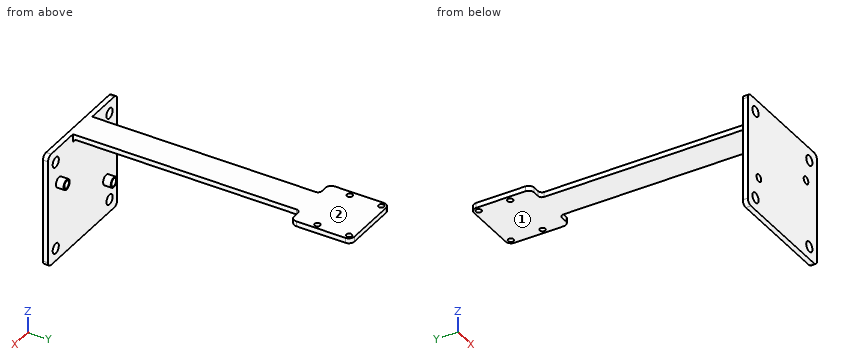
from build123d import *

# Parameters (mm, degrees)
SKETCH1_R           = 1.1
BOSS_EXTRUDE1_DEPTH = 2
FILLET1_R           = 2.2
FILLET2_R           = 2.2
FILLET3_R           = 2.2
FILLET5_R           = 2.2
FILLET6_R           = 1.5
FILLET7_R           = 1.5
SKETCH5_W           = 45
SKETCH5_H           = 45
SKETCH5_R           = 2
BOSS_EXTRUDE4_DEPTH = 2
FILLET17_R          = 2
FILLET18_R          = 2
FILLET19_R          = 2
FILLET20_R          = 2
FILLET21_R          = 1.5
SKETCH7_R           = 2
BOSS_EXTRUDE8_DEPTH = 5
SKETCH10_R          = 1.5
CUT_EXTRUDE4_DEPTH  = 6


with BuildPart() as part:
    # Sketch1 → Boss-Extrude1 (new body)
    with BuildSketch(Plane.XY):
        Polygon((6.25, 0), (6.25, -90), (18.75, -90), (18.75, 0), (25, 0), (25, 23.862), (0, 23.862), (0, 0), align=None)
        with Locations((2, 21.862)):
            Circle(SKETCH1_R, mode=Mode.SUBTRACT)
        with Locations((23, 21.862)):
            Circle(SKETCH1_R, mode=Mode.SUBTRACT)
        with Locations((2, 9.362)):
            Circle(SKETCH1_R, mode=Mode.SUBTRACT)
        with Locations((23, 9.362)):
            Circle(SKETCH1_R, mode=Mode.SUBTRACT)
    extrude(amount=BOSS_EXTRUDE1_DEPTH)

    # Fillet1
    fillet1_edges = [part.edges().sort_by_distance(p)[0] for p in [
        (0, 0, 1),
    ]]
    fillet(fillet1_edges, radius=FILLET1_R)

    # Fillet2
    fillet2_edges = [part.edges().sort_by_distance(p)[0] for p in [
        (0, 23.862, 1),
    ]]
    fillet(fillet2_edges, radius=FILLET2_R)

    # Fillet3
    fillet3_edges = [part.edges().sort_by_distance(p)[0] for p in [
        (25, 23.862, 1),
    ]]
    fillet(fillet3_edges, radius=FILLET3_R)

    # Fillet5
    fillet5_edges = [part.edges().sort_by_distance(p)[0] for p in [
        (25, 0, 1),
    ]]
    fillet(fillet5_edges, radius=FILLET5_R)

    # Fillet6
    fillet6_edges = [part.edges().sort_by_distance(p)[0] for p in [
        (18.75, 0, 1),
    ]]
    fillet(fillet6_edges, radius=FILLET6_R)

    # Fillet7
    fillet7_edges = [part.edges().sort_by_distance(p)[0] for p in [
        (6.25, 0, 1),
    ]]
    fillet(fillet7_edges, radius=FILLET7_R)

    # Sketch5 → Boss-Extrude4 (add)
    with BuildSketch(Plane.XZ.offset(90)):
        with Locations((12.5, -20.5)):
            Rectangle(SKETCH5_W, SKETCH5_H)
        with Locations((-5, -3)):
            Circle(SKETCH5_R, mode=Mode.SUBTRACT)
        with Locations((-5, -38)):
            Circle(SKETCH5_R, mode=Mode.SUBTRACT)
        with Locations((30, -3)):
            Circle(SKETCH5_R, mode=Mode.SUBTRACT)
        with Locations((30, -38)):
            Circle(SKETCH5_R, mode=Mode.SUBTRACT)
    extrude(amount=BOSS_EXTRUDE4_DEPTH)

    # Fillet17
    fillet17_edges = [part.edges().sort_by_distance(p)[0] for p in [
        (35, -91, 2),
    ]]
    fillet(fillet17_edges, radius=FILLET17_R)

    # Fillet18
    fillet18_edges = [part.edges().sort_by_distance(p)[0] for p in [
        (-10, -91, 2),
    ]]
    fillet(fillet18_edges, radius=FILLET18_R)

    # Fillet19
    fillet19_edges = [part.edges().sort_by_distance(p)[0] for p in [
        (-10, -91, -43),
    ]]
    fillet(fillet19_edges, radius=FILLET19_R)

    # Fillet20
    fillet20_edges = [part.edges().sort_by_distance(p)[0] for p in [
        (35, -91, -43),
    ]]
    fillet(fillet20_edges, radius=FILLET20_R)

    # Fillet21
    fillet21_edges = [part.edges().sort_by_distance(p)[0] for p in [
        (12.5, -90, 0),
    ]]
    fillet(fillet21_edges, radius=FILLET21_R)

    # Sketch7 → Boss-Extrude8 (add)
    with BuildSketch(Plane.XZ.offset(92)):
        with Locations((27.85, -12.25)):
            Circle(SKETCH7_R)
        with Locations((-2.85, -28.75)):
            Circle(SKETCH7_R)
    extrude(amount=-BOSS_EXTRUDE8_DEPTH)

    # Sketch10 → Cut-Extrude4 (cut, through all)
    with BuildSketch(Plane(origin=(0, -87, 0), x_dir=(1, 0, 0), z_dir=(0, 1, 0))):
        with Locations((27.85, 12.25)):
            Circle(SKETCH10_R)
        with Locations((-2.85, 28.75)):
            Circle(SKETCH10_R)
    extrude(amount=-CUT_EXTRUDE4_DEPTH, mode=Mode.SUBTRACT)


solid = part.part
Input: part model. Units: mm. Frame: model coordinates. Face numbers are marked on the shaded views. A direction names the side the tool comes from. Give positions to 0.01 mm unless a question says otherwise; leave off trailing zeros. Order: outer loops, then holes, each group sorted by start corner. A loop starts at its lowest first (then second) coordinate and runs counter-clockwise, first axis right, second up.
Q1. Contact query for flat-ended pins moving along their axis: pin 1 Ø1 at (y, z) = (11.5, 1) entering from +X; pin 2 Ø20 at (x, y) = (15, -30) entering from -Z; pin 3 Ø3 at (x, z) = (-2.5, -29) entering from +Y. Output: stop coordinate, or through.
Checked values:
pin 1: stops at x = 25
pin 2: stops at z = 0
pin 3: stops at y = -87
Q2. Section A-A on z = -38. Output: boundary loops of the cut face in (x, y), and give its area (3 significant figures).
Checked values:
outline: (-10, -92) - (-7, -92) - (-7, -90) - (-10, -90) - close; (-3, -92) - (28, -92) - (28, -90) - (-3, -90) - close; (32, -92) - (35, -92) - (35, -90) - (32, -90) - close
area: 74.0 mm2
Q3. Set-up query: the marked faces 1 and 2. Return all of +Z, -Z, +X, -X, +Y, -Y with unobstructed straight access to the full face (end or side cutting, diameter ignored); none if empty.
Checked values:
face 1: -Z, +X, -X, +Y
face 2: +Z, +X, -X, +Y, -Y
Q4. Section C-C on z = -28.75. Output: boundary loops of the cut face in (x, y).
Checked values:
outline: (-10, -92) - (-4.35, -92) - (-4.35, -87) - (-4.85, -87) - (-4.85, -90) - (-10, -90) - close; (-1.35, -92) - (35, -92) - (35, -90) - (-0.85, -90) - (-0.85, -87) - (-1.35, -87) - close
Q5. Section D-D on y = -79. Output: boundary loops of the cut face in (x, z).
Checked values:
outline: (6.25, 0) - (18.75, 0) - (18.75, 2) - (6.25, 2) - close
Q6. Ray query, probe 1 along Y at (x, z) = (2, 1.1); probe 2 along Z at (x, y) = (30, -90.7); probe 3 along X at (y, z) = (-90.75, -12.25). Return the intervals inside material, ascending.
Checked values:
probe 1: y = -92 to -90, 0.01 to 8.26, 10.46 to 20.76, 22.96 to 23.85
probe 2: z = -43 to -40, -36 to -5, -1 to 2
probe 3: x = -10 to 26.35, 29.35 to 35
Q7. Section B-B on x = 11. Output: boundary loops of the cut face in (y, z).
Checked values:
outline: (-92, -43) - (-90, -43) - (-90, -1.5) arc R1.5 cw to (-88.5, 0) - (23.86, 0) - (23.86, 2) - (-92, 2) - close
